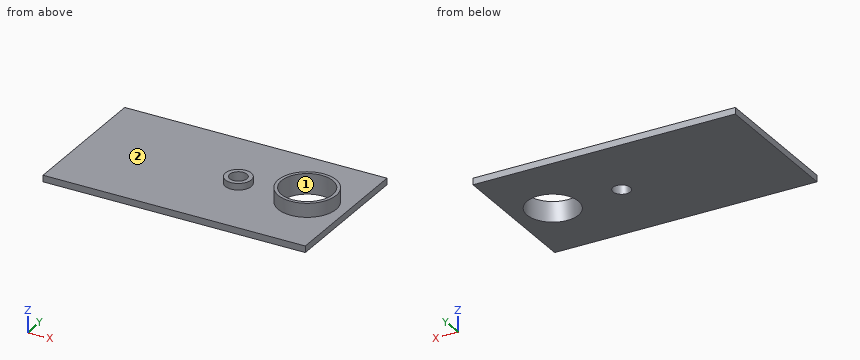
Autodesk Inventor part; units mm, degrees
ref_plane "YZ Plane" through (0, 0, 0) normal (1, 0, 0) x (0, 1, 0)
ref_plane "XZ Plane" through (0, 0, 0) normal (0, 1, 0) x (-1, 0, 0)
ref_plane "XY Plane" through (0, 0, 0) normal (0, 0, 1) x (1, 0, 0)
sketch "Sketch1" plane through (0, 0, 0) normal (0, 0, 1) x (1, 0, 0)
  line L0 (-14.5985, 9.3978) -> (106.6015, 9.3978)
  line L1 (106.6015, 9.3978) -> (106.6015, -56.8022)
  line L2 (106.6015, -56.8022) -> (-14.5985, -56.8022)
  line L3 (-14.5985, -56.8022) -> (-14.5985, 9.3978)
  circle A0 centre (88.6015, -23.7022) radius 11.9
  circle A1 centre (56.8015, -23.7022) radius 4
  point P0 (0, 0)
  dimension "d0" = 121.2
  dimension "d1" = 66.2
  dimension "d3" = 33.1
  dimension "d4" = 8
  dimension "d5" = 23.8
  dimension "d6" = 18
  dimension "d17" = 31.8
extrude "Extrusion1" add sketch "Sketch1" along normal mid plane 3
sketch "Sketch2" plane through (0, 0, 1.5) normal (0, 0, 1) x (1, 0, 0)
  circle A0 centre (56.8015, -23.7022) radius 4
  circle A1 centre (56.8015, -23.7022) radius 6
  point P0 (0, 0)
  dimension "d10" = 12
extrude "Extrusion2" add sketch "Sketch2" along normal blind 3
sketch "Sketch3" plane through (0, 0, 1.5) normal (0, 0, 1) x (1, 0, 0)
  circle A0 centre (88.6015, -23.7022) radius 11.9
  circle A1 centre (88.6015, -23.7022) radius 13.4
  point P0 (0, 0)
  dimension "d13" = 23.8
  dimension "d14" = 26.8
extrude "Extrusion3" add sketch "Sketch3" along normal blind 6.4
equation "\"d3\" = 0.5 * d1"
properties part number "Cover"
Read the model definition and answer for the solid it produces. Units are mm, in the model's axes. Face numbers are marked on the shaded views. Coordinates: 2 decimals unless noted, no trailing zeros. Loops run counter-clockwise (first coordinate to the right, second up) from the corner with the lowest first, then second, coordinate; pieces in that order, holes last. Notation, with made-up numbers: (-12, -31.5) - (19, -31.5) arc R23 ccw to (19, -4.5) - close; hole circle Ø8 at (-3.75, -8.5). An arc over 180 degrees is marked (long way). Answer in a Markdown table with one row per item.
Q1. Straight lines are drawn through the part: line 1 along Y through (x, z) = (88, 2); line 2 along Z through (x, y) = (30, -10); line 3 along X through (y, z) = (-26.5, 4.25). For each, find the intervals that lie inside material, in ascending order. Write a range as [from, to].
Here are the results:
| item | result |
|---|---|
| line 1 | y = [-37.09, -35.59], [-11.82, -10.32] |
| line 2 | z = [-1.5, 1.5] |
| line 3 | x = [51.49, 53.94], [59.66, 62.11], [75.5, 77.04], [100.17, 101.71] |
Q2. Find section A-A on y = -39.5. Write down the section's boundary in (x, z), plus the area to 3 significant figures.
Here are the results:
| item | result |
|---|---|
| outline | (-14.6, -1.5) - (106.6, -1.5) - (106.6, 1.5) - (-14.6, 1.5) - close |
| area | 364 mm^2 |
Q3. Find section C-C on z = 5.75. Write down the section's boundary in (x, y).
Here are the results:
| item | result |
|---|---|
| outline | circle Ø26.8 at (88.6, -23.7); hole circle Ø23.8 at (88.6, -23.7) |
Q4. Given P1, Ø21.5, axis at x = 88.6, y = -23.7, coming from the +Z side (3 decimals); P2, Ø20, axis at x = 65, y = -33.5, coming from the +Z side; P3, Ø1.5, axis at x = 28.5, y = -8, coming from the +Z side, each flat-ended and moving along its own axis, determine where each tip first touches the part or whether it passes through.
Here are the results:
| item | result |
|---|---|
| P1 | passes through |
| P2 | stops at z = 4.5 |
| P3 | stops at z = 1.5 |
Q5. The mould has two halves that part along Y. Classify the marked faces 1 and 2: pulls with the +Y half, pulls with the -Y half, needs draft (parallel to the pull), parting line crosses it, or undercut.
Here are the results:
| item | result |
|---|---|
| face 1 | undercut |
| face 2 | needs draft |
Q6. Find section B-B on x = 49. Write down the section's boundary in (y, z).
Here are the results:
| item | result |
|---|---|
| outline | (-56.8, -1.5) - (9.4, -1.5) - (9.4, 1.5) - (-56.8, 1.5) - close |
